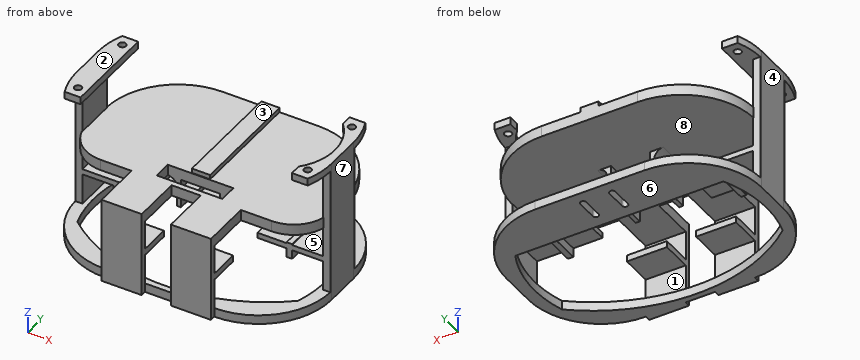
from build123d import *

# Parameters (mm, degrees)
SKETCH1_W                 = 140
SKETCH1_H                 = 100
BOSS_EXTRUDE1_DEPTH       = 5
SKETCH2_W                 = 4
SKETCH2_H                 = 52
BOSS_EXTRUDE2_DEPTH       = 70
SKETCH3_W                 = 12
SKETCH3_H                 = 52
BOSS_EXTRUDE3_DEPTH       = 4
SKETCH4_R                 = 2
CUT_EXTRUDE1_DEPTH        = 4
SKETCH5_W                 = 70
SKETCH5_H                 = 15
CUT_EXTRUDE3_DEPTH        = 169.347854159
FILLET1_R                 = 40
CUT_EXTRUDE6_DEPTH        = 10
SKETCH11_W                = 22
SKETCH11_H                = 41
BOSS_EXTRUDE6_DEPTH       = 3
SKETCH12_W                = 22
SKETCH12_H                = 6
BOSS_EXTRUDE7_DEPTH       = 30
SKETCH15_W                = 132.6
SKETCH15_H                = 76
BOSS_EXTRUDE8_DEPTH       = 6
FILLET2_R                 = 40
FILLET3_R                 = 20
CUT_EXTRUDE13_DEPTH       = 10
SKETCH25_W                = 10
SKETCH25_H                = 62.648578198
BOSS_EXTRUDE9_DEPTH       = 2.5
BOSS_EXTRUDE10_DEPTH      = 16
SKETCH27_W                = 21.5
SKETCH27_H                = 2.5
BOSS_EXTRUDE11_DEPTH      = 26
FILLET4_R                 = 5
SKETCH29_W                = 14
SKETCH29_H                = 10
CUT_EXTRUDE14_DEPTH       = 5
CUT_EXTRUDE15_DEPTH       = 5
SKETCH33_W                = 36
SKETCH33_H                = 3
BOSS_EXTRUDE12_DEPTH      = 22
BOSS_EXTRUDE13_DEPTH      = 5
BOSS_EXTRUDE13_DEPTH_BACK = 3.5
SKETCH34_W                = 22
SKETCH34_H                = 17
SKETCH34_W_2              = 3
SKETCH34_H_2              = 22
SKETCH35_W                = 5
SKETCH35_H                = 17
CUT_EXTRUDE16_DEPTH       = 139.021737418
SKETCH36_W                = 36.01199305
SKETCH36_H                = 10
CUT_EXTRUDE17_DEPTH       = 8


with BuildPart() as part:
    # Sketch1 → Boss-Extrude1 (new body)
    with BuildSketch(Plane.XY):
        Rectangle(SKETCH1_W, SKETCH1_H)
    extrude(amount=BOSS_EXTRUDE1_DEPTH)

    # Sketch2 → Boss-Extrude2 (add)
    with BuildSketch(Plane.XY.offset(5)):
        with Locations((-68, 0)):
            Rectangle(SKETCH2_W, SKETCH2_H)
        with Locations((68, 0)):
            Rectangle(SKETCH2_W, SKETCH2_H)
    extrude(amount=BOSS_EXTRUDE2_DEPTH)

    # Sketch3 → Boss-Extrude3 (add)
    with BuildSketch(Plane.XY.offset(75)):
        with Locations((-64, 0)):
            Rectangle(SKETCH3_W, SKETCH3_H)
        with Locations((64, 0)):
            Rectangle(SKETCH3_W, SKETCH3_H)
    extrude(amount=BOSS_EXTRUDE3_DEPTH)

    # Sketch4 → Cut-Extrude1 (cut)
    with BuildSketch(Plane.XY.offset(79)):
        with Locations((-63, 20)):
            Circle(SKETCH4_R)
        with Locations(Location((-63, -20, 0), (0, 0, 180))):
            Circle(SKETCH4_R)
        with Locations(Location((63, 20, 0), (0, 0, 180))):
            Circle(SKETCH4_R)
        with Locations((63, -20)):
            Circle(SKETCH4_R)
    extrude(amount=-CUT_EXTRUDE1_DEPTH, mode=Mode.SUBTRACT)

    # Sketch5 → Cut-Extrude3 (cut, through all)
    with BuildSketch(Plane.ZY.offset(70)):
        with Locations((40, 18.5)):
            Rectangle(SKETCH5_W, SKETCH5_H)
        with Locations((40, -18.5)):
            Rectangle(SKETCH5_W, SKETCH5_H)
    extrude(amount=-CUT_EXTRUDE3_DEPTH, mode=Mode.SUBTRACT)

    # Fillet1
    fillet1_edges = [part.edges().sort_by_distance(p)[0] for p in [
        (70, -50, 2.5),
        (70, 50, 2.5),
        (-70, 50, 2.5),
        (-70, -50, 2.5),
    ]]
    fillet(fillet1_edges, radius=FILLET1_R)

    # Sketch9 → Cut-Extrude6 (cut)
    with BuildSketch(Plane(origin=(0, 0, 0), x_dir=(-1, 0, 0), z_dir=(0, 0, -1))):
        with BuildLine():
            Line((-6.4, 42.595375442), (-6.4, 31.250081589))
            ThreePointArc((-6.4, 31.250081589), (-8, 29.650081589), (-9.6, 31.250081589))
            Line((-9.6, 31.250081589), (-9.6, 42.595375442))
            ThreePointArc((-9.6, 42.595375442), (-8, 44.195375442), (-6.4, 42.595375442))
        make_face()
        with BuildLine():
            Line((6.4, 42.595375442), (6.4, 31.250081589))
            ThreePointArc((6.4, 31.250081589), (8, 29.650081589), (9.6, 31.250081589))
            Line((9.6, 31.250081589), (9.6, 42.595375442))
            ThreePointArc((9.6, 42.595375442), (8, 44.195375442), (6.4, 42.595375442))
        make_face()
    extrude(amount=-CUT_EXTRUDE6_DEPTH, mode=Mode.SUBTRACT)

    # Sketch11 → Boss-Extrude6 (add)
    with BuildSketch(Plane.XZ.offset(50)):
        with Locations((-19, 20.5)):
            Rectangle(SKETCH11_W, SKETCH11_H)
        with Locations((19, 20.5)):
            Rectangle(SKETCH11_W, SKETCH11_H)
    extrude(amount=BOSS_EXTRUDE6_DEPTH)

    # Sketch12 → Boss-Extrude7 (add)
    with BuildSketch(Plane.XZ.offset(53)):
        with Locations((-19, 44)):
            Rectangle(SKETCH12_W, SKETCH12_H)
        with Locations((19, 44)):
            Rectangle(SKETCH12_W, SKETCH12_H)
    extrude(amount=-BOSS_EXTRUDE7_DEPTH)

    # Sketch15 → Boss-Extrude8 (add)
    with BuildSketch(Plane.XY.offset(47)):
        with Locations((0, 12)):
            Rectangle(SKETCH15_W, SKETCH15_H)
    extrude(amount=-BOSS_EXTRUDE8_DEPTH)

    # Fillet2
    # the kernel refuses this fillet: 40 mm, written as the material it takes off along each edge
    with BuildSketch(Plane(origin=(66.3, 50, 146.968745116), x_dir=(0, -1, 0), z_dir=(0, 0, -1))) as fillet2_piece_1_section:
        with BuildLine():
            CenterArc((40, 39.987498046), FILLET2_R, 180, 88.567456262)
            Line((0, 39.987498046), (0, 0))
            Line((0, 0), (39, 0))
        make_face()
    fillet2_piece_1 = extrude(amount=105.968745116, mode=Mode.PRIVATE)
    fillet2_piece_1 = split(fillet2_piece_1, bisect_by=Plane(origin=(65.992272223, 15.649976228, 75), z_dir=(0, 0, -1)), keep=Keep.TOP, mode=Mode.PRIVATE)
    add(fillet2_piece_1, mode=Mode.SUBTRACT)
    with BuildSketch(Plane(origin=(-66.3, 50, 146.968745116), x_dir=(0, -1, 0), z_dir=(0, 0, -1))) as fillet2_piece_2_section:
        with BuildLine():
            CenterArc((40, -39.987498046), FILLET2_R, 91.432543738, 88.567456262)
            Line((0, -39.987498046), (0, 0))
            Line((0, 0), (39, 0))
        make_face()
    fillet2_piece_2 = extrude(amount=105.968745116, mode=Mode.PRIVATE)
    fillet2_piece_2 = split(fillet2_piece_2, bisect_by=Plane(origin=(-65.992272223, 15.649976228, 75), z_dir=(0, 0, -1)), keep=Keep.TOP, mode=Mode.PRIVATE)
    add(fillet2_piece_2, mode=Mode.SUBTRACT)

    # Fillet3
    # the kernel refuses this fillet: 20 mm, written as the material it takes off along each edge
    with BuildSketch(Plane(origin=(66.3, -26, 47), x_dir=(0, 1, 0), z_dir=(0, 0, -1))) as fillet3_piece_1_section:
        with BuildLine():
            CenterArc((20, -19.364916731), FILLET3_R, 104.477512186, 75.522487814)
            Line((0, -19.364916731), (0, 0))
            Line((0, 0), (15, 0))
        make_face()
    fillet3_piece_1 = extrude(amount=54.412291828, mode=Mode.PRIVATE)
    fillet3_piece_1 = split(fillet3_piece_1, bisect_by=Plane(origin=(64.996360144, -14.682849628, 5), z_dir=(0, 0, 1)), keep=Keep.TOP, mode=Mode.PRIVATE)
    add(fillet3_piece_1, mode=Mode.SUBTRACT)
    with BuildSketch(Plane(origin=(-66.3, -26, 47), x_dir=(1, 0, 0), z_dir=(0, 0, -1))) as fillet3_piece_2_section:
        with BuildLine():
            CenterArc((19.364916731, -20), FILLET3_R, 90, 75.522487814)
            Line((0, -15), (0, 0))
            Line((0, 0), (19.364916731, 0))
        make_face()
    fillet3_piece_2 = extrude(amount=54.412291828, mode=Mode.PRIVATE)
    fillet3_piece_2 = split(fillet3_piece_2, bisect_by=Plane(origin=(-52.725602454, -25.185189276, 5), z_dir=(0, 0, 1)), keep=Keep.TOP, mode=Mode.PRIVATE)
    add(fillet3_piece_2, mode=Mode.SUBTRACT)

    # Sketch24 → Cut-Extrude13 (cut)
    with BuildSketch(Plane(origin=(0, 0, 0), x_dir=(-1, 0, 0), z_dir=(0, 0, -1))):
        with BuildLine():
            Line((57.127807538, 23.220760353), (-57.127807538, 23.220760353))
            ThreePointArc((-57.127807538, 23.220760353), (-63.480824357, -0.367653581), (-60.579297228, -24.623688601))
            ThreePointArc((-60.579297228, -24.623688601), (0, -46.779239647), (60.579297228, -24.623688601))
            ThreePointArc((60.579297228, -24.623688601), (63.401945013, -0.373343922), (57.127807538, 23.220760353))
        make_face()
    extrude(amount=-CUT_EXTRUDE13_DEPTH, mode=Mode.SUBTRACT)

    # Sketch25 → Boss-Extrude9 (add)
    with BuildSketch(Plane.XY.offset(47)):
        with Locations((0, 18.675710901)):
            Rectangle(SKETCH25_W, SKETCH25_H)
    extrude(amount=BOSS_EXTRUDE9_DEPTH)

    # Sketch26 → Boss-Extrude10 (add)
    with BuildSketch(Plane(origin=(0, 0, 41), x_dir=(-1, 0, 0), z_dir=(0, 0, -1))):
        Polygon((-10.75, -13), (-10.75, -11), (-10.75, 11), (-10.75, 13), (-13, 13), (-13, -13), align=None)
        Polygon((10.75, 11), (10.75, -11), (10.75, -13), (13, -13), (13, 13), (10.75, 13), align=None)
    extrude(amount=BOSS_EXTRUDE10_DEPTH)

    # Sketch27 → Boss-Extrude11 (add)
    with BuildSketch(Plane(origin=(0, 13, 0), x_dir=(1, 0, 0), z_dir=(0, 1, 0))):
        with Locations((0, -34.75)):
            Rectangle(SKETCH27_W, SKETCH27_H)
    extrude(amount=-BOSS_EXTRUDE11_DEPTH)

    # Fillet4
    fillet4_edges = [part.edges().sort_by_distance(p)[0] for p in [
        (13, 0, 41),
        (-13, 0, 41),
    ]]
    fillet(fillet4_edges, radius=FILLET4_R)

    # Sketch29 → Cut-Extrude14 (cut)
    with BuildSketch(Plane(origin=(0, 0, 33.5), x_dir=(-1, 0, 0), z_dir=(0, 0, -1))):
        with Locations((-3.75, -8)):
            Rectangle(SKETCH29_W, SKETCH29_H)
    extrude(amount=-CUT_EXTRUDE14_DEPTH, mode=Mode.SUBTRACT)

    # Sketch30 → Cut-Extrude15 (cut)
    with BuildSketch(Plane(origin=(0, 0, 75), x_dir=(-1, 0, 0), z_dir=(0, 0, -1))):
        with BuildLine():
            Line((-58, 20), (-58, -20))
            ThreePointArc((-58, -20), (-65.783189716, 0), (-58, 20))
        make_face()
    extrude(amount=-CUT_EXTRUDE15_DEPTH, mode=Mode.SUBTRACT)

    # Sketch33 → Boss-Extrude12 (add)
    with BuildSketch(Plane(origin=(0, 11, 0), x_dir=(1, 0, 0), z_dir=(0, 1, 0))):
        with Locations((-48, -23.5)):
            Rectangle(SKETCH33_W, SKETCH33_H)
        with Locations((48, -22.973655472)):
            Rectangle(SKETCH33_W, SKETCH33_H)
    extrude(amount=-BOSS_EXTRUDE12_DEPTH)

    # Sketch34 → Boss-Extrude13 (add, two sides: drawn at the far end of the back side and taken through both)
    with BuildSketch(Plane(origin=(0, 0, 21.473655472), x_dir=(-1, 0, 0), z_dir=(0, 0, -1)).offset(-BOSS_EXTRUDE13_DEPTH_BACK)):
        with Locations((19, -41.5)):
            Rectangle(SKETCH34_W, SKETCH34_H)
        with Locations((47.5, 0)):
            Rectangle(SKETCH34_W_2, SKETCH34_H_2)
        with Locations((-19, -41.5)):
            Rectangle(SKETCH34_W, SKETCH34_H)
        with Locations((-47.5, 0)):
            Rectangle(SKETCH34_W_2, SKETCH34_H_2)
    extrude(amount=BOSS_EXTRUDE13_DEPTH + BOSS_EXTRUDE13_DEPTH_BACK)

    # Sketch35 → Cut-Extrude16 (cut, through all)
    with BuildSketch(Plane.ZY.offset(30)):
        with Locations((18.973655472, -41.5)):
            Rectangle(SKETCH35_W, SKETCH35_H)
    extrude(amount=-CUT_EXTRUDE16_DEPTH, mode=Mode.SUBTRACT)

    # Sketch36 → Cut-Extrude17 (cut)
    with BuildSketch(Plane(origin=(0, 0, 41), x_dir=(-1, 0, 0), z_dir=(0, 0, -1))):
        with Locations((0.005996525, -18)):
            Rectangle(SKETCH36_W, SKETCH36_H)
    extrude(amount=-CUT_EXTRUDE17_DEPTH, mode=Mode.SUBTRACT)


solid = part.part
Could you check a few things on this model? Use its own coordinates, in mm. Face numbers are marked on the shaded views. A direction names the side the tool comes from. Coordinates: 2 decimals unless noted, no trailing zeros. Loops run counter-clockwise (first coordinate to the right, second up) from the corner with the lowest first, then second, coordinate; pieces in that order, holes last. Notation, with made-up numbers: (72.25, 17) -> (88.25, 17) arc R31 ccw to (88.25, 45) -> close; hole circle Ø5 at (61.5, -38). An arc over 180 degrees is marked (long way). Answer in a Markdown table with one row per item.
(1) If I drill on probe 1 along Z at (x, y) = (14, -48); probe 2 along Z at (x, y) = (55, 7); probe 3 along Y at (x, z) = (63, 77.9), over which ranges is the centre line in solid material (lowest first)?
Results found:
| item | result |
|---|---|
| probe 1 | z = 0 to 5, 21.47 to 24.97, 41 to 47 |
| probe 2 | z = 21.47 to 24.47, 41 to 47 |
| probe 3 | y = -26 to -22, -18 to -12.53, 12.53 to 18, 22 to 26 |
(2) For the marked faces 1, 2, 3, 4 and 5, which set-ups out of +Z, -Z, +X, -X, +Y, -Y let a thin tool reach every point of the face, with its end or its side?
Results found:
| item | result |
|---|---|
| face 1 | +X, -X, +Y |
| face 2 | +Z, +X, -X, +Y, -Y |
| face 3 | +Z, +Y, -Y |
| face 4 | +Z, -Z, -X, +Y, -Y |
| face 5 | +Y, -Y |
(3) Imagine slicing it at A-A (z = 11.5). List the corners of the cut face in (x, y) for me.
Results found:
| item | result |
|---|---|
| outline | (-70, -10) arc R40 ccw to (-69.99, -11) -> (-66, -11) -> (-66, 11) -> (-69.99, 11) arc R40 ccw to (-70, 10) -> close; (-30, -53) -> (-8, -53) -> (-8, -50) -> (-30, -50) -> close; (8, -53) -> (30, -53) -> (30, -50) -> (8, -50) -> close; (66, -11) -> (69.99, -11) arc R40 ccw to (70, -10) -> (70, 10) arc R40 ccw to (69.99, 11) -> (66, 11) -> close |
(4) Imagine slicing it at B-B (z = 68). List the corners of the cut face in (x, y) for me, plus the area to 3 significant figures.
Results found:
| item | result |
|---|---|
| outline | (-70, -10) arc R40 ccw to (-69.99, -11) -> (-66, -11) -> (-66, 11) -> (-69.99, 11) arc R40 ccw to (-70, 10) -> close; (66, -11) -> (69.99, -11) arc R40 ccw to (70, -10) -> (70, 10) arc R40 ccw to (69.99, 11) -> (66, 11) -> close |
| area | 176 mm^2 |
(5) Thinking about a two-plate mould opening in Z: for the marked faces 6, 7 and 8, which applies, released by +Z, released by -Z, zero draft, split by the parting line, or undercut?
Results found:
| item | result |
|---|---|
| face 6 | released by -Z |
| face 7 | zero draft |
| face 8 | undercut |
(6) Will these pins go through, and if not, where does the flat tip stop? pin 1 Ø6 at (x, y) = (-37.5, -39) entering from +Z; pin 2 Ø1.1 at (x, y) = (11.5, -5.5) entering from -Z; pin 3 Ø5 at (x, z) = (22.5, 15) entering from +Y; pin 4 Ø8 at (y, z) = (-34, 35) entering from -X.
Results found:
| item | result |
|---|---|
| pin 1 | stops at z = 5 |
| pin 2 | stops at z = 25 |
| pin 3 | stops at y = -50 |
| pin 4 | passes through |
(7) Imagine slicing it at C-C (x = 22). List the corners of the cut face in (y, z) for me.
Results found:
| item | result |
|---|---|
| outline | (-53, 0) -> (-44.17, 0) -> (-44.17, 5) -> (-50, 5) -> (-50, 21.47) -> (-33, 21.47) -> (-33, 24.97) -> (-50, 24.97) -> (-50, 41) -> (50, 41) -> (50, 47) -> (-53, 47) -> close; (23.22, 0) -> (50, 0) -> (50, 5) -> (23.22, 5) -> close |
(8) Imagine slicing it at D-D (y = -42). List the corners of the cut face in (x, z) for me (3 decimals), plus the area to 3 significant figures.
Results found:
| item | result |
|---|---|
| outline | (-54, 0) -> (-29.575, 0) -> (-29.575, 5) -> (-54, 5) -> close; (-30, 21.474) -> (-8, 21.474) -> (-8, 24.974) -> (-30, 24.974) -> close; (-30, 41) -> (-8, 41) -> (-8, 47) -> (-30, 47) -> close; (8, 21.474) -> (30, 21.474) -> (30, 24.974) -> (8, 24.974) -> close; (8, 41) -> (30, 41) -> (30, 47) -> (8, 47) -> close; (29.575, 0) -> (54, 0) -> (54, 5) -> (29.575, 5) -> close |
| area | 662 mm^2 |
